Autodesk Inventor part; units mm, degrees
ref_plane "YZ Plane" through (0, 0, 0) normal (1, 0, 0) x (0, 1, 0)
ref_plane "XZ Plane" through (0, 0, 0) normal (0, 1, 0) x (-1, 0, 0)
ref_plane "XY Plane" through (0, 0, 0) normal (0, 0, 1) x (1, 0, 0)
sketch "Sketch1" plane through (0, 0, 0) normal (0, 1, 0) x (-1, 0, 0)
  circle A0 centre (0, 0) radius 4
  dimension "d0" = 8
extrude "Extrusion1" add sketch "Sketch1" along normal blind 15
sketch "Sketch2" plane through (0, 15, 0) normal (0, 1, 0) x (1, 0, 0)
  circle A0 centre (0, 0) radius 3
  dimension "d3" = 6
extrude "Extrusion2" cut sketch "Sketch2" against normal blind 13
sketch "Sketch3" plane through (0, 0, 0) normal (1, 0, 0) x (0, 1, 0)
  line L0 (15, -4) -> (15, 4)
  circle A0 centre (4, 0) radius 2
  line L1 (0, -4) -> (0, 4)
  point P0 (0, 0)
  dimension "d8" = 4
  dimension "d9" = 4
extrude "Extrusion3" cut sketch "Sketch3" against normal through all both and the other way through all
sketch "Sketch9" plane through (0, 15, 0) normal (0, 1, 0) x (1, 0, 0)
  circle A0 centre (0, 0) radius 40
  dimension "d47" = 80
extrude "Extrusion8" add sketch "Sketch9" along normal blind 4
sketch "Sketch10" plane through (0, 19, 0) normal (0, 1, 0) x (1, 0, 0)
  circle A0 centre (0, 0) radius 3
  circle A1 centre (-33, 0) radius 2.25
  arc A2 (3, 0) -> (-3, 0) centre (0, 0) ccw
  line L0 (0, 0) -> (-40, 0)
  circle A3 centre (0, 0) radius 4
  arc A4 (-31.2581, -10.5797) -> (-24.7914, -21.7805) centre (0, 0) ccw
  arc A5 (-29.8813, -8.0067) -> (-31.2581, -10.5797) centre (-29.3637, -9.9385) ccw
  arc A6 (-24.7914, -21.7805) -> (-21.8746, -21.8746) centre (-23.2889, -20.4604) ccw
  arc A7 (-9.0928, -4.1619) -> (-8.1507, -5.7937) centre (0, 0) ccw
  line L1 (-8.3666, -8.3666) -> (-21.8746, -21.8746)
  line L2 (-11.429, -3.0624) -> (-29.8813, -8.0067)
  arc A8 (-8.3666, -8.3666) -> (-8.1507, -5.7937) centre (-9.7808, -6.9524) ccw
  arc A9 (-9.0928, -4.1619) -> (-11.429, -3.0624) centre (-10.9114, -4.9942) ccw
  arc A10 (-6.4667, -32.3602) -> (6.4667, -32.3602) centre (0, 0) ccw
  line L3 (-3.0624, -11.429) -> (-8.0067, -29.8813)
  arc A11 (-0.9421, -9.9555) -> (-3.0624, -11.429) centre (-1.1305, -11.9466) ccw
  line L4 (3.0624, -11.429) -> (8.0067, -29.8813)
  arc A12 (-0.9421, -9.9555) -> (0.9421, -9.9555) centre (0, 0) ccw
  arc A13 (3.0624, -11.429) -> (0.9421, -9.9555) centre (1.1305, -11.9466) ccw
  arc A14 (6.4667, -32.3602) -> (8.0067, -29.8813) centre (6.0748, -30.399) ccw
  arc A15 (-8.0067, -29.8813) -> (-6.4667, -32.3602) centre (-6.0748, -30.399) ccw
  arc A16 (24.7914, -21.7805) -> (31.2581, -10.5797) centre (0, 0) ccw
  line L5 (8.3666, -8.3666) -> (21.8746, -21.8746)
  arc A17 (8.1507, -5.7937) -> (8.3666, -8.3666) centre (9.7808, -6.9524) ccw
  line L6 (11.429, -3.0624) -> (29.8813, -8.0067)
  arc A18 (8.1507, -5.7937) -> (9.0928, -4.1619) centre (0, 0) ccw
  arc A19 (11.429, -3.0624) -> (9.0928, -4.1619) centre (10.9114, -4.9942) ccw
  arc A20 (31.2581, -10.5797) -> (29.8813, -8.0067) centre (29.3637, -9.9385) ccw
  arc A21 (21.8746, -21.8746) -> (24.7914, -21.7805) centre (23.2889, -20.4604) ccw
  arc A22 (31.2581, 10.5797) -> (24.7914, 21.7805) centre (0, 0) ccw
  line L7 (11.429, 3.0624) -> (29.8813, 8.0067)
  arc A23 (9.0928, 4.1619) -> (11.429, 3.0624) centre (10.9114, 4.9942) ccw
  line L8 (8.3666, 8.3666) -> (21.8746, 21.8746)
  arc A24 (9.0928, 4.1619) -> (8.1507, 5.7937) centre (0, 0) ccw
  arc A25 (8.3666, 8.3666) -> (8.1507, 5.7937) centre (9.7808, 6.9524) ccw
  arc A26 (24.7914, 21.7805) -> (21.8746, 21.8746) centre (23.2889, 20.4604) ccw
  arc A27 (29.8813, 8.0067) -> (31.2581, 10.5797) centre (29.3637, 9.9385) ccw
  arc A28 (6.4667, 32.3602) -> (-6.4667, 32.3602) centre (0, 0) ccw
  line L9 (3.0624, 11.429) -> (8.0067, 29.8813)
  arc A29 (0.9421, 9.9555) -> (3.0624, 11.429) centre (1.1305, 11.9466) ccw
  line L10 (-3.0624, 11.429) -> (-8.0067, 29.8813)
  arc A30 (0.9421, 9.9555) -> (-0.9421, 9.9555) centre (0, 0) ccw
  arc A31 (-3.0624, 11.429) -> (-0.9421, 9.9555) centre (-1.1305, 11.9466) ccw
  arc A32 (-6.4667, 32.3602) -> (-8.0067, 29.8813) centre (-6.0748, 30.399) ccw
  arc A33 (8.0067, 29.8813) -> (6.4667, 32.3602) centre (6.0748, 30.399) ccw
  arc A34 (-24.7914, 21.7805) -> (-31.2581, 10.5797) centre (0, 0) ccw
  line L11 (-8.3666, 8.3666) -> (-21.8746, 21.8746)
  arc A35 (-8.1507, 5.7937) -> (-8.3666, 8.3666) centre (-9.7808, 6.9524) ccw
  line L12 (-11.429, 3.0624) -> (-29.8813, 8.0067)
  arc A36 (-8.1507, 5.7937) -> (-9.0928, 4.1619) centre (0, 0) ccw
  arc A37 (-11.429, 3.0624) -> (-9.0928, 4.1619) centre (-10.9114, 4.9942) ccw
  arc A38 (-31.2581, 10.5797) -> (-29.8813, 8.0067) centre (-29.3637, 9.9385) ccw
  arc A39 (-21.8746, 21.8746) -> (-24.7914, 21.7805) centre (-23.2889, 20.4604) ccw
  point P0 (-31.8756, -8.541)
  point P1 (-23.3345, -23.3345)
  point P2 (-9.6593, -2.5882)
  point P3 (-7.0711, -7.0711)
  dimension "d54" = 4.5
  dimension "d62" = 2
  dimension "d63" = 2
  dimension "d66" = 360
extrude "Extrusion9" cut sketch "Sketch10" against normal through all contours A0 | A1 L0 | L0 A1 | A5 L2 A9 A7 A8 L1 A6 A4 | A15 L3 A11 A12 A13 L4 A14 A10 | A21 L5 A17 A18 A19 L6 A20 A16 | A27 L7 A23 A24 A25 L8 A26 A22 | A33 L9 A29 A30 A31 L10 A32 A28 | A39 L11 A35 A36 A37 L12 A38 A34
properties part number "trục quay"
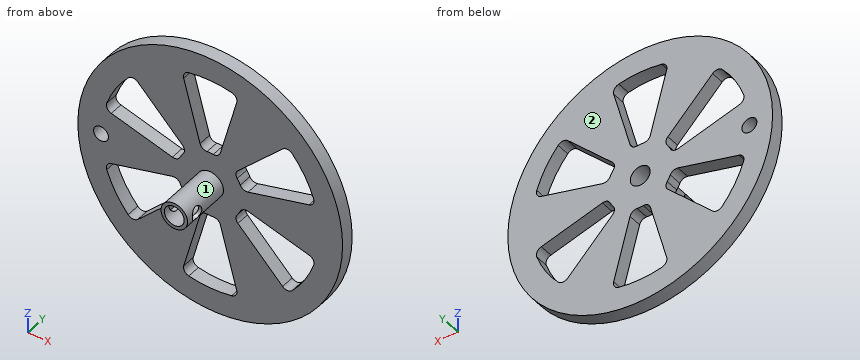
Model file for the job. Use its own axes, mm. Face numbers are marked on the shaded views. A direction names the side the tool comes from. Give positions to 0.01 mm unless a question says otherwise; leave off trailing zeros. Order: outer loops, then holes, each group sorted by start corner. A loop starts at its lowest first (then second) coordinate and runs counter-clockwise, first axis right, second up. Notation, with made-up numbers: (82.5, -28.75) - (98.5, -28.75) arc R29 cw to (98.5, 7.25) - close; hole circle Ø6 at (-30.5, -25.75). An arc over 180 degrees is marked (long way). Write item = value, one per line. Start each with the question number.
1. Cut at B-B, the plane z = -12.5. List the corners of the cut face in (x, y), and give its area (3 significant figures).
2. Cut at A-A, the plane x = -33.5. List the corners of the cut face in (y, z).
3. Drop flat-ended pins along their axis: P1, Ø6.5, axis at y = 4, z = 0, coming from the -X side; P2, Ø1.5, axis at x = -4, z = -5.5, coming from the -Y side. Give the stop position or say it passes through.
4. Cut at D-D, the plane y = 9.25. List the corners of the cut face in (x, z).
5. Cut at C-C, the plane z = 0. List the corners of the cut face in (x, y).
6. Which spindle directions (+Z, -Z, +X, -X, +Y, -Y) get a long thin tool onto all of the face, cutting with end or side? Do the marked faces 1 and 2. Say none if no direction does.
7. Probe line 1 along X through (y, z) = (17.55, 0); line 2 along Z through (x, y) = (-18, 16.75); line 3 along Y through (x, z) = (-3.25, 0). List the from-to ranges inside material, lowest first.
Taken from the geometry:
q1.outline = (-38, 15) - (-30.54, 15) - (-30.54, 19) - (-38, 19) - close; (-12.5, 15) - (-3.35, 15) - (-3.35, 19) - (-12.5, 19) - close; (3.35, 15) - (12.5, 15) - (12.5, 19) - (3.35, 19) - close; (30.54, 15) - (38, 15) - (38, 19) - (30.54, 19) - close
q1.area = 133 mm²
q2.outline = (15, -21.86) - (19, -21.86) - (19, -2.19) - (15, -2.19) - close; (15, 2.19) - (19, 2.19) - (19, 21.86) - (15, 21.86) - close
q3.P1 = -4
q3.P2 = 15
q4.outline = circle Ø8 at (0, 0); hole circle Ø6 at (0, 0)
q5.outline = (-40, 15) - (-35.25, 15) - (-35.25, 19) - (-40, 19) - close; (-30.75, 15) - (-4, 15) - (-4, 6) - (-3, 6) - (-3, 19) - (-30.75, 19) - close; (-4, 0) - (-3, 0) - (-3, 2) - (-4, 2) - close; (3, 0) - (4, 0) - (4, 2) - (3, 2) - close; (3, 6) - (4, 6) - (4, 15) - (40, 15) - (40, 19) - (3, 19) - close
q6.face_1 = -Y
q6.face_2 = +Z, -Z, +X, -X, +Y
q7.line_1 = -40 to -35.25, -30.75 to -3, 3 to 40
q7.line_2 = -35.72 to -18, -4.82 to 4.82, 18 to 35.72
q7.line_3 = 0 to 2, 6 to 19
